Build history of the part. All positions in model axes, mm. A direction names the side the tool comes from. Give positions to 0.01 mm unless a question says otherwise; leave off trailing zeros. Order: outer loops, then holes, each group sorted by start corner. A loop starts at its lowest first (then second) coordinate and runs counter-clockwise, first axis right, second up. Notation, with made-up numbers: (52.25, 12.5) - (103.25, 12.5) arc R7 cw to (103.25, 17.5) - close; hole circle Ø1 at (-2, 48.5). An arc over 180 degrees is marked (long way). One line per item, written item: value.
Autodesk Inventor part; units mm, degrees
ref_plane "YZ Plane" through (0, 0, 0) normal (1, 0, 0) x (0, 1, 0)
ref_plane "XZ Plane" through (0, 0, 0) normal (0, 1, 0) x (-1, 0, 0)
ref_plane "XY Plane" through (0, 0, 0) normal (0, 0, 1) x (1, 0, 0)
sketch "Sketch1" plane through (0, 0, 0) normal (0, 0, 1) x (1, 0, 0)
  line L0 (0, 0) -> (50.8, 0)
  line L1 (50.8, 0) -> (50.8, 25.4)
  line L2 (50.8, 25.4) -> (0, 25.4)
  line L3 (0, 25.4) -> (0, 0)
  line L4 (49.149, 23.749) -> (1.651, 23.749)
  line L5 (1.651, 23.749) -> (1.651, 1.651)
  line L6 (1.651, 1.651) -> (49.149, 1.651)
  line L7 (49.149, 1.651) -> (49.149, 23.749)
  line L8 (49.149, 23.749) -> (1.651, 1.651) construction
  line L9 (1.651, 23.749) -> (49.149, 1.651) construction
  point P0 (25.4, 12.7)
  dimension "d0" = 1.651
  dimension "d1" = 25.4
  dimension "d2" = 50.8
  dimension "d3" = 1.651
  dimension "d4" = 1.651
  dimension "d5" = 1.651
extrude "Extrusion1" add sketch "Sketch1" along normal blind 76.2
sketch "Sketch2" plane through (0, 25.4, 0) normal (0, 1, 0) x (1, 0, 0)
  circle A0 centre (25.4, -38.1) radius 9.525
  line L0 (50.8, 0) -> (50.8, -76.2)
  line L1 (50.8, -76.2) -> (0, -76.2)
  point P0 (0, 0)
  dimension "d8" = 19.05
  dimension "d9" = 25.4
  dimension "d10" = 38.1
extrude "Extrusion2" cut sketch "Sketch2" against normal blind 76.2
sketch "Sketch4" plane through (0, 25.4, 0) normal (0, 1, 0) x (1, 0, 0)
  circle A0 centre (25.1665, -14.2875) radius 2.5797
  circle A1 centre (25.4, -38.1) radius 9.525
  circle A2 centre (25.4, -38.1) radius 23.8136 construction
  circle A3 centre (4.661, -26.396) radius 2.5797
  circle A4 centre (4.8945, -50.2085) radius 2.5797
  circle A5 centre (25.6335, -61.9125) radius 2.5797
  circle A6 centre (46.139, -49.804) radius 2.5797
  circle A7 centre (45.9055, -25.9915) radius 2.5797
  point P0 (0, 0)
  dimension "d31" = 23.8125
  dimension "d32" = 5.1594
  dimension "d35" = 360
extrude "Extrusion4" cut sketch "Sketch4" against normal blind 76.2 contours A0 | A3 | A4 | A5 | A6 | A7
equation "\"d3\" = d0"
equation "\"d4\" = d0"
equation "\"d5\" = d0"
properties part number "hub attachment"
(1) Slice it at D-D, the plane x = 17. Give the cut face in (y, z).
Completed:
outline: (0, 0) - (1.65, 0) - (1.65, 33.61) - (0, 33.61) - close; (0, 42.59) - (1.65, 42.59) - (1.65, 76.2) - (0, 76.2) - close; (23.75, 0) - (25.4, 0) - (25.4, 33.61) - (23.75, 33.61) - close; (23.75, 42.59) - (25.4, 42.59) - (25.4, 76.2) - (23.75, 76.2) - close
(2) Pull direction X, two halves, no side cores. Call faces 3 (the face through (31, 25.4, 46)), 4 (the face through (0, 13, 38)), 5 (the face through (50.8, 13, 38)), 6 (the face through (48.366, 0.837, 25.217)): +X half, -X half, draft (parallel to the pull), parting line (faces both ways), or undercut.
Completed:
face 3: draft
face 4: -X half
face 5: +X half
face 6: undercut
(3) Slice it at C-C, the plane x = 11. Give the cut face in (y, z), and give its area (3 significant figures).
Completed:
outline: (0, 0) - (1.65, 0) - (1.65, 76.2) - (0, 76.2) - close; (23.75, 0) - (25.4, 0) - (25.4, 76.2) - (23.75, 76.2) - close
area: 252 mm²
(4) Slice it at A-A, the plane z = 38.1. Give the cut face in (x, y) (3 decimals).
Completed:
outline: (0, 0) - (15.875, 0) - (15.875, 1.651) - (1.651, 1.651) - (1.651, 23.749) - (15.875, 23.749) - (15.875, 25.4) - (0, 25.4) - close; (34.925, 0) - (50.8, 0) - (50.8, 25.4) - (34.925, 25.4) - (34.925, 23.749) - (49.149, 23.749) - (49.149, 1.651) - (34.925, 1.651) - close
(5) Slice it at B-B, the plane y = 17.25. Give the cut face in (x, z), and give its area (3 significant figures).
Completed:
outline: (0, 0) - (1.65, 0) - (1.65, 76.2) - (0, 76.2) - close; (49.15, 0) - (50.8, 0) - (50.8, 76.2) - (49.15, 76.2) - close
area: 252 mm²
(6) Drill centre lines: line 1 (Z direction, x = 25.4, y = 0.9) (3 decimals); line 2 (Y direction, x = 3, z = 60); line 3 (X direction, y = 6.25, z = 23). Where is each one in solid material? Low to high.
Completed:
line 1: 0 to 11.718, 16.857 to 28.575, 47.625 to 59.343, 64.482 to 76.2
line 2: 0 to 1.65, 23.75 to 25.4
line 3: 0 to 1.65, 49.15 to 50.8
(7) 3-axis set-ups, long thin cutter, end or side, ignore diameter. For faces 1 (the face through (20, 1.651, 29)), 2 (the face through (31, 0, 46)): which of +Z, -Z, +X, -X, +Y, -Y reach the whole face in a straight line?
Completed:
face 1: +Z, -Z
face 2: +Z, -Z, +X, -X, -Y
